Autodesk Inventor part; units mm, degrees
ref_plane "YZ Plane" through (0, 0, 0) normal (1, 0, 0) x (0, 1, 0)
ref_plane "XZ Plane" through (0, 0, 0) normal (0, 1, 0) x (-1, 0, 0)
ref_plane "XY Plane" through (0, 0, 0) normal (0, 0, 1) x (1, 0, 0)
sketch "Sketch1" plane through (0, 0, 0) normal (0, 1, 0) x (-1, 0, 0)
  line L0 (0, 0) -> (-12.7, 0)
  line L1 (-12.7, 0) -> (-12.7, 304.8)
  line L2 (-12.7, 304.8) -> (0, 304.8)
  line L3 (0, 304.8) -> (0, 0)
  dimension "d0" = 304.8
  dimension "d1" = 12.7
extrude "Extrusion1" add sketch "Sketch1" along normal blind 25.4
sketch "Sketch2" plane through (12.7, 0, 304.8) normal (1, 0, 0) x (0, 0, -1)
  circle A0 centre (279.4, 12.7) radius 3.175
  line L0 (304.8, 0) -> (304.8, 25.4)
  line L1 (0, 25.4) -> (304.8, 25.4)
  circle A1 centre (25.4, 12.7) radius 3.175
  line L2 (0, 0) -> (0, 25.4)
  line L3 (304.8, 0) -> (0, 0)
  dimension "d4" = 6.35
  dimension "d5" = 25.4
  dimension "d6" = 12.7
  dimension "d7" = 6.35
  dimension "d8" = 25.4
  dimension "d9" = 12.7
extrude "Extrusion2" cut sketch "Sketch2" against normal through all contours A0 | A1
properties part number "arm3"
Build history of the part. All positions in model axes, mm. Round coordinates to 2 decimals unless told otherwise and drop trailing zeros. Loops run counter-clockwise (first coordinate to the right, second up) from the corner with the lowest first, then second, coordinate; pieces in that order, holes last. Notation, with made-up numbers: M -10,37 L 24,37 A11 cw 24,55 Z; hole C -20,15 d1. An arc over 180 degrees is marked long. Answer as CSV lines item,"result".
1. Cut at A-A on y = 12.7. Write the cut outline in (x, z) (3 decimals), then the cut area to 3 significant figures.
Resolved:
outline,"M 0,0 L 12.7,0 L 12.7,22.225 L 0,22.225 Z; M 0,28.575 L 12.7,28.575 L 12.7,276.225 L 0,276.225 Z; M 0,282.575 L 12.7,282.575 L 12.7,304.8 L 0,304.8 Z"
area,"3,710 mm²"
2. Cut at B-B on z = 279.4. Write the cut outline in (x, y) (3 decimals), then the cut area to 3 significant figures.
Resolved:
outline,"M 0,0 L 12.7,0 L 12.7,9.525 L 0,9.525 Z; M 0,15.875 L 12.7,15.875 L 12.7,25.4 L 0,25.4 Z"
area,"242 mm²"
3. Two-plate mould, pull along Y, no slides. Class faces 1 (the flat face through (12.7, 13, 150)), 2 (the cylindrical face through (6.44, 10.77, 281.92)), 3 (the cylindrical face through (6.44, 11.48, 22.47)), 4 (the flat face through (6, 25.4, 155)): released by +Y, released by -Y, zero draft, split by the parting line, or undercut.
Resolved:
face 1,"zero draft"
face 2,"undercut"
face 3,"undercut"
face 4,"released by +Y"
4. Wall check: probe 1 along Y at (x, z) = (9.5, 25.4) (3 decimals); probe 2 along Y at (x, z) = (9.5, 23). Give the ranges that are in metal, low to high. Write a range as [from, to].
Resolved:
probe 1,"y = [0, 9.525], [15.875, 25.4]"
probe 2,"y = [0, 10.62], [14.78, 25.4]"
5. Flat gauge pin, fed straight in: P1, Ø3, axis at x = 6, y = 16.5, coming from the -Z side. Where does the tip first touch, or does it go through?
Resolved:
P1,"stops at z = 0"
